```python
from build123d import *

# Parameters (mm, degrees)
BOSS_EXTRUDE1_DEPTH = 7


with BuildPart() as part:
    # Sketch1 → Boss-Extrude1 (new body)
    with BuildSketch(Plane(origin=(0, 0, 0), x_dir=(1, 0, 0), z_dir=(0, 1, 0))):
        with BuildLine():
            Line((52.5, -100), (-52.5, -100))
            ThreePointArc((-52.5, -100), (-63.106601718, -95.606601718), (-67.5, -85))
            Line((-67.5, -85), (-67.5, 100))
            ThreePointArc((-67.5, 100), (0, 167.5), (67.5, 100))
            Line((67.5, 100), (67.5, -85))
            ThreePointArc((67.5, -85), (63.106601718, -95.606601718), (52.5, -100))
        make_face()
    extrude(amount=BOSS_EXTRUDE1_DEPTH)


solid = part.part
```
Read the model definition and answer for the solid it produces. Units are mm, in the model's axes. Coordinates: 2 decimals unless noted, no trailing zeros. Write each loop counter-clockwise with the first axis right and the second up, starting at its lowest first coordinate (ties: lowest second). Pieces come first, ordered by that corner, then holes. Notation, with made-up numbers: (84.5, -12.5) - (111.5, -12.5) arc R23 ccw to (111.5, 24.5) - close; hole circle Ø6 at (-11.75, -11.75). An arc over 180 degrees is marked (long way). Answer as a JSON object with one key per item and string values. Group by question number.
1. A cutting plane is placed at C-C (z = -130.5). Determine the outline of the cut face in (x, y).
2. A cutting plane is placed at A-A (y = 5.25). Determine the outline of the cut face in (x, z), plus the area to 3 significant figures.
3. This flat-tipped pin is pushed along its axis until it touches: P1, Ø3, axis at x = -4.5, y = 4, coming from the -Z side. Where does it stop, or does it pass through?
4. A cutting plane is placed at B-B (x = 57.5). Determine the outline of the cut face in (y, z), plus the area to 3 significant figures.
5. Consider L1, parallel to Z at x = -1.5, y = 5; L2, parallel to Z at x = 3, y = 1; L3, parallel to X at y = 6.75, z = -132.5. Determine where each line is inside the solid, lowest interval first. Write a range as [from, to].
Worked out:
{
 "1": {"outline": "(-60.22, 0) - (60.22, 0) - (60.22, 7) - (-60.22, 7) - close"},
 "2": {"outline": "(-67.5, -100) arc R67.5 ccw to (67.5, -100) - (67.5, 85) arc R15 ccw to (52.5, 100) - (-52.5, 100) arc R15 ccw to (-67.5, 85) - close", "area": "34,100 mm²"},
 "3": {"P1": "stops at z = -167.43"},
 "4": {"outline": "(0, -135.36) - (7, -135.36) - (7, 99.14) - (0, 99.14) - close", "area": "1,640 mm²"},
 "5": {"L1": "z = [-167.48, 100]", "L2": "z = [-167.43, 100]", "L3": "x = [-59.16, 59.16]"}
}
